from build123d import *

# Parameters (mm, degrees)
SKETCH1_R           = 2.299249708
BOSS_EXTRUDE1_DEPTH = 2
BOSS_EXTRUDE2_DEPTH = 25
CUT_EXTRUDE1_DEPTH  = 5
CUT_EXTRUDE2_DEPTH  = 122.722871427


with BuildPart() as part:
    # Sketch1 → Boss-Extrude1 (new body)
    with BuildSketch(Plane.XY):
        with BuildLine():
            Line((-50.442352941, -22.916302521), (-22.442352941, -22.916302521))
            ThreePointArc((-22.442352941, -22.916302521), (-11.414384755, 0.055729293), (11.557647059, 11.083697479))
            Line((11.557647059, 11.083697479), (11.557647059, 39.083697479))
            Line((11.557647059, 39.083697479), (-22.442352941, 73.083697479))
            Line((-22.442352941, 73.083697479), (-50.442352941, 73.083697479))
            ThreePointArc((-50.442352941, 73.083697479), (-61.477304412, 50.118648949), (-84.442352941, 39.083697479))
            Line((-84.442352941, 39.083697479), (-84.442352941, 11.083697479))
            Line((-84.442352941, 11.083697479), (-91.513420753, 4.012629667))
            Line((-91.513420753, 4.012629667), (-57.513420753, -29.987370333))
            Line((-57.513420753, -29.987370333), (-50.442352941, -22.916302521))
        make_face()
        with Locations((-36.442352941, 25.083697479)):
            Circle(SKETCH1_R, mode=Mode.SUBTRACT)
    extrude(amount=BOSS_EXTRUDE1_DEPTH)

    # Sketch2 → Boss-Extrude2 (add)
    with BuildSketch(Plane.XY.offset(2)):
        with BuildLine():
            Line((11.557647059, 11.083697479), (11.557647059, 39.083697479))
            Line((11.557647059, 39.083697479), (3.941530535, 46.699814003))
            Line((3.941530535, 46.699814003), (3.144174906, 45.902458373))
            Line((3.144174906, 45.902458373), (10.470077714, 38.576555565))
            Line((10.470077714, 38.576555565), (10.361931826, 12.13145892))
            ThreePointArc((10.361931826, 12.13145892), (-12.239549802, 0.88089434), (-23.490114382, -21.720587289))
            Line((-23.490114382, -21.720587289), (-49.935211027, -21.828733177))
            Line((-49.935211027, -21.828733177), (-50.442352941, -22.916302521))
            Line((-50.442352941, -22.916302521), (-22.442352941, -22.916302521))
            ThreePointArc((-22.442352941, -22.916302521), (-11.407401471, 0.048746009), (11.557647059, 11.083697479))
        make_face()
        with BuildLine():
            Line((-22.442352941, 73.083697479), (-50.442352941, 73.083697479))
            ThreePointArc((-50.442352941, 73.083697479), (-61.477304412, 50.118648949), (-84.442352941, 39.083697479))
            Line((-84.442352941, 39.083697479), (-84.442352941, 11.083697479))
            Line((-84.442352941, 11.083697479), (-83.354783597, 11.590839393))
            Line((-83.354783597, 11.590839393), (-83.246637709, 38.035936038))
            ThreePointArc((-83.246637709, 38.035936038), (-60.64515608, 49.286500618), (-49.394591501, 71.887982247))
            Line((-49.394591501, 71.887982247), (-22.949494855, 71.996128135))
            Line((-22.949494855, 71.996128135), (-15.623592047, 64.670225326))
            Line((-15.623592047, 64.670225326), (-14.826236418, 65.467580955))
            Line((-14.826236418, 65.467580955), (-22.442352941, 73.083697479))
        make_face()
    extrude(amount=-BOSS_EXTRUDE2_DEPTH)

    # Sketch3 → Cut-Extrude1 (cut)
    with BuildSketch(Plane(origin=(0, 0, 0), x_dir=(-1, 0, 0), z_dir=(0, 0, -1))):
        Polygon((31.712662704, -21.754212985), (31.712662704, -22.916302521), (41.712662704, -22.916302521), (41.712662704, -21.79510748), (41.712662704, -21.572636028), (31.712662704, -21.531741532), align=None)
        Polygon((-10.395557523, 29.813387716), (-11.557647059, 29.813387716), (-11.557647059, 19.813387716), (-10.436452018, 19.813387716), (-10.213980565, 19.813387716), (-10.17308607, 29.813387716), align=None)
        Polygon((41.172043178, 71.921607943), (41.172043178, 73.083697479), (31.172043178, 73.083697479), (31.172043178, 71.962502438), (31.172043178, 71.740030985), (41.172043178, 71.69913649), align=None)
        Polygon((83.280263405, 20.354007242), (84.442352941, 20.354007242), (84.442352941, 30.354007242), (83.3211579, 30.354007242), (83.098686448, 30.354007242), (83.057791952, 20.354007242), align=None)
    extrude(amount=CUT_EXTRUDE1_DEPTH, mode=Mode.SUBTRACT)

    # Sketch4 → Cut-Extrude2 (cut, through all)
    with BuildSketch(Plane(origin=(25.320672269, 25.320672269, 0), x_dir=(0.707106781, -0.707106781, 0), z_dir=(0.707106781, 0.707106781, 0))):
        with BuildLine():
            Line((-87.346107905, 12.335462167), (-87.346107905, 23))
            Line((-87.346107905, 23), (0.335132962, 23))
            Line((0.335132962, 23), (0.335132962, 12.335462167))
            add(Edge.make_bspline(
                [(-87.346107905, 12.335462167), (-59.446253938, 22.367177976), (-27.564721006, 22.367177976), (0.335132962, 12.335462167)],
                knots=[0, 0, 0, 0, 1, 1, 1, 1], degree=3))
        make_face()
    extrude(amount=-CUT_EXTRUDE2_DEPTH, mode=Mode.SUBTRACT)


solid = part.part
CAD build for the part. Positions are in the model's coordinates, mm. A direction names the side the tool comes from. Round coordinates to 2 decimals unless told otherwise and drop trailing zeros. Loops run counter-clockwise (first coordinate to the right, second up) from the corner with the lowest first, then second, coordinate; pieces in that order, holes last. Notation, with made-up numbers: M 42,85.25 L 62,85.25 A19 ccw 62,113.25 Z; hole C 6,42.5 d7. An arc over 180 degrees is marked long. One line per question, with ' | ' between items. Start each with the question number.
Item 1: Two-plate mould, pull along X, no slides. Class faces 1 (the flat face through (-36, 73.084, -8)), 2 (the flat face through (-19.338, 68.384, -9.464)), 3 (the flat face through (-84.442, 25, -8)): pulls with the +X half, pulls with the -X half, needs draft (parallel to the pull), parting line crosses it, or undercut.
Item 2: Cut at A-A, the plane z = -11. Write the cut outline in (x, y).
Item 3: Cut at B-B, the plane z = -3. State how many separate pieces and enclosed holes the cut face has, plus the area to 3 significant figures.
Item 4: Pin check, flat tips, straight feed: pin 1 Ø8 at (x, y) = (-59, 8) entering from -Z; pin 2 Ø8 at (x, z) = (-15, -13) entering from +Y; pin 3 Ø3 at (x, z) = (-7.5, -9.5) entering from -Y. Stop position of each tip, or through.
Item 5: Wall check: line 1 (Y direction, x = -31, z = -1.75); line 2 (Y direction, x = -28, z = -2); line 3 (Z direction, x = -60.5, y = 4). Give the ranges that are in metal, low to high.
Item 6: Which spindle directions (+Z, -Z, +X, -X, +Y, -Y) get a long thin tool onto all of the face, cutting with end or side? Do faces 4 (the flat face through (-37, -22.916, -8)), 5 (the cylindrical face through (-35.206, 27.022, 0.986)). Say none if no direction does.
Responses:
1) face 1: needs draft | face 2: undercut | face 3: pulls with the -X half
2) outline: M -84.44,11.08 L -83.35,11.59 L -83.25,38.04 A39.71 ccw -49.39,71.89 L -22.95,72 L -15.62,64.67 L -14.83,65.47 L -22.44,73.08 L -50.44,73.08 A38.48 cw -84.44,39.08 Z; M -50.44,-22.92 L -22.44,-22.92 A38.48 cw 11.56,11.08 L 11.56,39.08 L 3.94,46.7 L 3.14,45.9 L 10.47,38.58 L 10.36,12.13 A39.71 ccw -23.49,-21.72 L -49.94,-21.83 Z
3) separate pieces: 6 | enclosed holes: 0 | area: 224 mm²
4) pin 1: stops at z = 0 | pin 2: stops at y = 69.64 | pin 3: stops at y = 2.26
5) line 1: y = -22.92 to -21.75, 71.96 to 73.08 | line 2: y = -22.92 to -21.74, 71.98 to 73.08 | line 3: z = 0 to 2
6) face 4: +Z, -Z, +X, -Y | face 5: +Z, -Z
